Here's how the part is built. I have some questions about the finished solid (model axes, mm). Face numbers are marked on the shaded views. A direction names the side the tool comes from. Coordinates: 2 decimals unless noted, no trailing zeros. Order: outer loops, then holes, each group sorted by start corner. A loop starts at its lowest first (then second) coordinate and runs counter-clockwise, first axis right, second up. Notation, with made-up numbers: M 13.5,54 L 35.5,54 A18 ccw 35.5,74 Z; hole C 53,-12 d5. An arc over 180 degrees is marked long. Answer as CSV lines item,"result". Start each with the question number.
```python
from build123d import *

# Parameters (mm, degrees)
F1_DEPTH = 50.8
F2_R     = 12.7
F3_R     = 6.35
F4_DEPTH = 101.601
F5_W     = 20.32
F5_H     = 38.1
F6_DEPTH = 88.9


with BuildPart() as f1:
    # F0 (on Front) → F1 (new body, symmetric)
    with BuildSketch(Plane.XZ):
        with BuildLine():
            Line((-3.81, 98.3185720786), (-3.81, 9.4185720786))
            ThreePointArc((-3.81, 9.4185720786), (0, -10.16), (3.81, 9.4185720786))
            Line((3.81, 9.4185720786), (3.81, 98.3185720786))
            Line((3.81, 98.3185720786), (-3.81, 98.3185720786))
        make_face()
    extrude(amount=F1_DEPTH, both=True)

    # F2
    f2_edges = [f1.edges().sort_by_distance(p)[0] for p in [
        (0, -50.8, 98.318572),
        (0, 50.8, 98.318572),
    ]]
    fillet(f2_edges, radius=F2_R)

    # F3 (on face) → F4 (cut, through all)
    with BuildSketch(Plane(origin=(0, 50.8, 0), x_dir=(-1, 0, 0), z_dir=(0, 1, 0))):
        Circle(F3_R)
    extrude(amount=-F4_DEPTH, mode=Mode.SUBTRACT)

    # F5 (on face) → F6 (cut, symmetric)
    with BuildSketch(Plane(origin=(-3.81, 0, 0), x_dir=(0, -1, 0), z_dir=(-1, 0, 0))):
        with Locations((40.64, -9.6314279214)):
            Rectangle(F5_W, F5_H)
        Polygon((10.16, 9.4185720786), (-10.16, 9.4185720786), (-10.16, -20.9424663335), (-10.16, -22.940389812), (10.16, -22.940389812), align=None)
        Polygon((-30.48, 9.4185720786), (-50.8, 9.4185720786), (-50.8, -9.6314279214), (-50.8, -22.1083164215), (-30.48, -22.1083164215), align=None)
    extrude(amount=F6_DEPTH, both=True, mode=Mode.SUBTRACT)


solid = f1.part
```
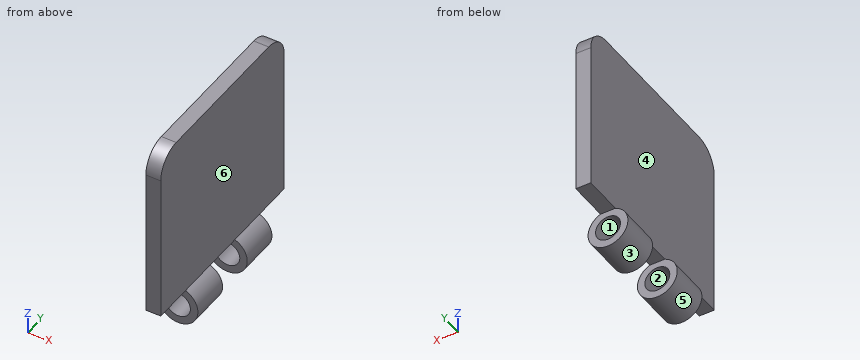
1) Suppose I cut it at B-B on x = 0. Please give me the cut outline in (y, z), plus the area to 3 significant figures.
2) Will these pins go through, and if not, where does the flat tip stop? pin 1 Ø2 at (y, z) = (-29.5, 24) entering from +X; pin 2 Ø11.5 at (x, z) = (0, 0) entering from -Y; pin 3 Ø6 at (x, y) = (2, -45) entering from -Z; pin 4 Ø10 at (x, z) = (-7, 77.5) entering from +Y.
3) Suppose I cut it at A-A on z = 0. Please give me the cut outline in (x, y), plus the area to 3 significant figures.
4) If we mould it in two halves opening along X, with no side actions, what happens to the marked faces 1, 2, 3 and 4? For each: released by +X, released by -X, zero draft, split by the parting line, or undercut.
5) Suppose I cut it at D-D on y = -28. Please give me the cut outline in (x, z), plus the area to 3 significant figures.
6) Suppose I cut it at C-C on x = -7.75. Please give me the cut outline in (y, z).
7) I need wall thicknesses on line 1 (Y direction, x = 5.5, z = -5); line 2 (X direction, y = 14.5, z = 0.5); line 3 (X direction, y = -14.5, z = 76.5). Which ranges of each line are inside material? Lowest first, please. Write a range as [from, to].
8) Which directions (+Z, -Z, +X, -X, +Y, -Y) give clear straight access to the entire face, cutting with the end or side of a thin tool? Please do the marked faces 5 and 6.
Output:
1,outline,"M -50.8,9.42 L -30.48,9.42 L -30.48,6.35 L -10.16,6.35 L -10.16,9.42 L 10.16,9.42 L 10.16,6.35 L 30.48,6.35 L 30.48,9.42 L 50.8,9.42 L 50.8,85.62 A12.7 ccw 38.1,98.32 L -38.1,98.32 A12.7 ccw -50.8,85.62 Z; M -30.48,-10.16 L -10.16,-10.16 L -10.16,-6.35 L -30.48,-6.35 Z; M 10.16,-10.16 L 30.48,-10.16 L 30.48,-6.35 L 10.16,-6.35 Z"
1,area,"9,240 mm²"
2,pin 1,"x = 3.81"
2,pin 2,"through"
2,pin 3,"z = 9.42"
2,pin 4,"y = 50.8"
3,outline,"M -10.16,-30.48 L -6.35,-30.48 L -6.35,-10.16 L -10.16,-10.16 Z; M -10.16,10.16 L -6.35,10.16 L -6.35,30.48 L -10.16,30.48 Z; M 6.35,-30.48 L 10.16,-30.48 L 10.16,-10.16 L 6.35,-10.16 Z; M 6.35,10.16 L 10.16,10.16 L 10.16,30.48 L 6.35,30.48 Z"
3,area,"310 mm²"
4,face 1,"undercut"
4,face 2,"undercut"
4,face 3,"split by the parting line"
4,face 4,"released by -X"
5,outline,"M -3.81,9.42 A10.16 ccw long 3.81,9.42 L 3.81,98.32 L -3.81,98.32 Z; hole C 0,0 d12.7"
5,area,"871 mm²"
6,outline,"M -30.48,-6.57 L -10.16,-6.57 L -10.16,6.57 L -30.48,6.57 Z; M 10.16,-6.57 L 30.48,-6.57 L 30.48,6.57 L 10.16,6.57 Z"
7,line 1,"[-30.48, -10.16], [10.16, 30.48]"
7,line 2,"[-10.15, -6.33], [6.33, 10.15]"
7,line 3,"[-3.81, 3.81]"
8,face 5,"+Y, -Y"
8,face 6,"+Z, +X, +Y, -Y"
